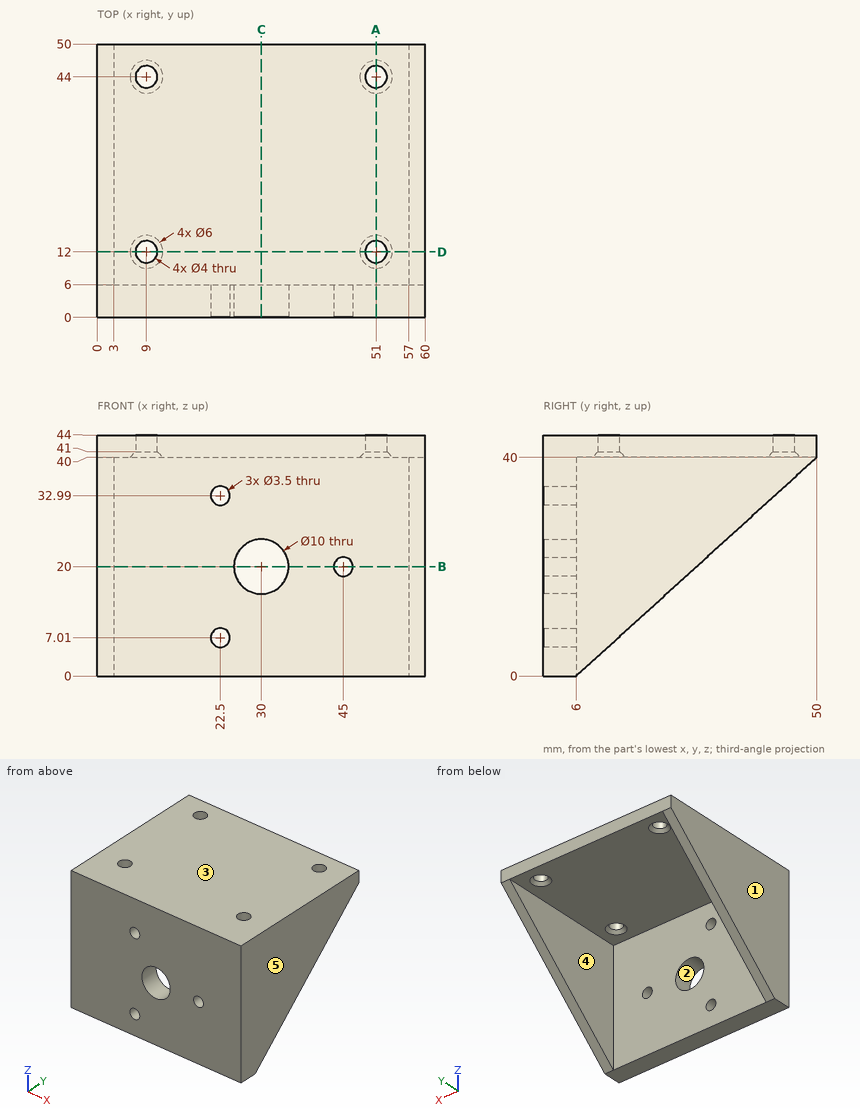
For this review, use the dimensioned drawing (mm, ordinates from the lowest corner) and the shaded views. A direction names the side the tool comes from. Give positions to 0.01 mm unless a question says otherwise; leave off trailing zeros. Loops run counter-clockwise (first coordinate to the right, second up) from the corner with the lowest first, then second, coordinate; pieces in that order, holes last. Notation, with made-up numbers: (2.5, -10) -> (6.5, -10) arc R28 cw to (6.5, 15) -> close; hole circle Ø11 at (-14, 3). An arc over 180 degrees is marked (long way). One line per question, with ' | ' between items. Start each with the question number.
(1) We need section A-A (x = 51). State the section outline as (y, z) points.
(2) We need section B-B (z = 20). State the section outline as (x, y) points, and give its area (3 significant figures).
(3) For the marked faces 4 and 5, list the 3-axis set-ups (+Z, -Z, +X, -X, +Y, -Y) from which the entire face can be reached by the end or side of a thin tool; tool diameter is ignored.
(4) Insertion check: P1, Ø20, axis at x = 23, z = 21, coming from the +Y side; P2, Ø1.5, axis at x = 37.5, y = 33.5, coming from the -Z side. Each pin has a flat end and moves straight along its axis. Give the tip position at first contact, or say it passes through.
(5) For line 1 (Y direction, x = 9, z = 43); line 2 (Z direction, x = 22.5, y = 1.9); line 3 (X direction, y = 44, z = 43.35), list the stretches that pass through material, from the lowest coordinate up.
(6) Draft analysis for pull direction Z (two halves, no side actions). For the marked faces 1, 2 and 3, state which applies: +Z half, -Z half, draft (parallel to the pull), parting line (faces both ways), or undercut.
(7) We need section C-C (x = 30). State the section outline as (y, z) points.
(8) We need section D-D (y = 12). State the section outline as (x, z) points (1 decimal).
The answers:
1) outline: (0, 0) -> (6, 0) -> (6, 40) -> (9, 40) -> (10, 41) -> (10, 44) -> (0, 44) -> close; (14, 41) -> (15, 40) -> (41, 40) -> (42, 41) -> (42, 44) -> (14, 44) -> close; (46, 41) -> (47, 40) -> (50, 40) -> (50, 44) -> (46, 44) -> close
2) outline: (0, 0) -> (25, 0) -> (25, 6) -> (3, 6) -> (3, 28) -> (0, 28) -> close; (35, 0) -> (43.25, 0) -> (43.25, 6) -> (35, 6) -> close; (46.75, 0) -> (60, 0) -> (60, 28) -> (57, 28) -> (57, 6) -> (46.75, 6) -> close | area: 411 mm^2
3) face 4: -Z, +Y | face 5: +Z, -Z, +X, +Y, -Y
4) P1: stops at y = 6 | P2: stops at z = 40
5) line 1: y = 0 to 10, 14 to 42, 46 to 50 | line 2: z = 0 to 5.26, 8.76 to 31.24, 34.74 to 44 | line 3: x = 0 to 7, 11 to 49, 53 to 60
6) face 1: draft | face 2: undercut | face 3: +Z half
7) outline: (0, 0) -> (6, 0) -> (6, 15) -> (0, 15) -> close; (0, 25) -> (6, 25) -> (6, 40) -> (50, 40) -> (50, 44) -> (0, 44) -> close
8) outline: (0, 5.5) -> (3, 5.5) -> (3, 40) -> (6, 40) -> (7, 41) -> (7, 44) -> (0, 44) -> close; (11, 41) -> (12, 40) -> (48, 40) -> (49, 41) -> (49, 44) -> (11, 44) -> close; (53, 41) -> (54, 40) -> (57, 40) -> (57, 5.5) -> (60, 5.5) -> (60, 44) -> (53, 44) -> close
